Read the model definition and answer for the solid it produces. Units are mm, in the model's axes. Face numbers are marked on the shaded views. Coordinates: 2 decimals unless noted, no trailing zeros. Order: outer loops, then holes, each group sorted by start corner. A loop starts at its lowest first (then second) coordinate and runs counter-clockwise, first axis right, second up. Notation, with made-up numbers: (-18.75, 8) -> (23.25, 8) arc R22 ccw to (23.25, 45) -> close; hole circle Ø4 at (85.25, 1.25). An arc over 180 degrees is marked (long way). Answer in a Markdown table with one row per item.
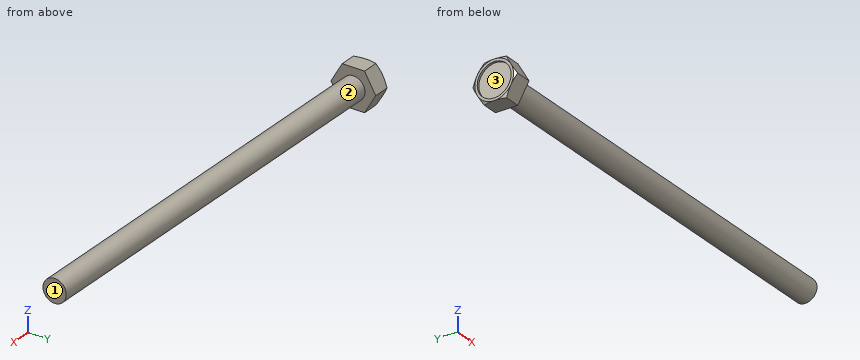
from build123d import *

# Parameters (mm, degrees)
SKETCH2_R     = 2.915704388
HEX_DIE_DEPTH = 2.3
SKETCH4_R     = 2.1875
INDENT_DEPTH  = 0.2875


with BuildPart() as part:
    # BodySke → Base-Revolve (revolve)
    with BuildSketch(Plane.XY):
        Polygon((2.3, 1.5), (2.3, 2.886836028), (0.223339885, 2.886836028), (0, 2.5), (0, 0), (57.3, 0), (57.3, 1.5), align=None)
    revolve(axis=Axis((-25.4, 0, 0), (1, 0, 0)))

    # Sketch2 → Hex-Die (cut)
    with BuildSketch(Plane(origin=(0, 0, 0), x_dir=(0, 0, -1), z_dir=(1, 0, 0))):
        Circle(SKETCH2_R)
        Polygon((-2.5, 1.443375679), (0, 2.886751359), (2.5, 1.443375679), (2.5, -1.443375679), (0, -2.886751359), (-2.5, -1.443375679), align=None, mode=Mode.SUBTRACT)
    extrude(amount=HEX_DIE_DEPTH, mode=Mode.SUBTRACT)

    # Sketch4 → Indent (cut)
    with BuildSketch(Plane(origin=(0, 0, 0), x_dir=(0, 0, -1), z_dir=(1, 0, 0))):
        Circle(SKETCH4_R)
    extrude(amount=INDENT_DEPTH, mode=Mode.SUBTRACT)


solid = part.part
Q1. For a pull along Y with two mould halves and no side action, classify the marked faces 1, 2 and 3 as pulls with the +Y half, pulls with the -Y half, needs draft (parallel to the pull), parting line crosses it, or undercut.
Outcome:
| item | result |
|---|---|
| face 1 | needs draft |
| face 2 | parting line crosses it |
| face 3 | undercut |
Q2. Consider line 1 (X direction, y = 2.45, z = -0.1); line 2 (X direction, y = 0.3, z = 0.5); line 3 (Y direction, x = 0.2, z = 0). Determine where each line is inside the solid, lowest interval first.
Outcome:
| item | result |
|---|---|
| line 1 | 0 to 2.3 |
| line 2 | 0.29 to 57.3 |
| line 3 | -2.85 to -2.19, 2.19 to 2.85 |
Q3. The part is cut by section A-A (x = 20). Write down the section's boundary in (y, z), then the cut area to 3 significant figures.
Outcome:
| item | result |
|---|---|
| outline | circle Ø3 at (0, 0) |
| area | 7.07 mm² |
Q4. Given pin 1 (1.3 mm diameter, centred on y = 0.5, z = 0.5, fed in from -X); pin 2 (1 mm diameter, centred on y = 1, z = 1.5, fed in from -X); pin 3 (1.5 mm diameter, centred on x = 42.5, y = 1, fed in from +Z); pin 4 (2 mm diameter, centred on x = 24, z = 0.5, fed in from +Y), each flat-ended and moving along its own axis, determine where each tip first touches the part or whether it passes through.
Outcome:
| item | result |
|---|---|
| pin 1 | x = 0.29 |
| pin 2 | x = 0 |
| pin 3 | z = 1.48 |
| pin 4 | y = 1.5 |
